```python
from build123d import *

# Parameters (mm, degrees)
SKETCH_2_R               = 72.5
EXTRUDE_1_DEPTH          = 2
CUT_EXTRUDE_1_DEPTH      = 103.549987811
CUT_EXTRUDE_1_DEPTH_BACK = 103.549987811
SKETCH_3_R               = 1.1


with BuildPart() as part:
    # 草图2 → 凸台-拉伸1 (new body)
    with BuildSketch(Plane(origin=(0, 0, 0), x_dir=(1, 0, 0), z_dir=(0, 1, 0))):
        with Locations(Location((0, 0, 0), (0, 0, 270))):
            Circle(SKETCH_2_R)
    extrude(amount=EXTRUDE_1_DEPTH)

    # 草图3 → 切除-拉伸1 (cut, two sides: drawn at the far end of the back side and taken through both)
    with BuildSketch(Plane.XZ.offset(-CUT_EXTRUDE_1_DEPTH_BACK)):
        with Locations(Location((32, 60, 0), (0, 0, 270))):
            Circle(SKETCH_3_R)
        with Locations(Location((-32, 60, 0), (0, 0, 270))):
            Circle(SKETCH_3_R)
        with Locations(Location((-32, -26, 0), (0, 0, 270))):
            Circle(SKETCH_3_R)
        with Locations(Location((32, -26, 0), (0, 0, 270))):
            Circle(SKETCH_3_R)
    extrude(amount=CUT_EXTRUDE_1_DEPTH + CUT_EXTRUDE_1_DEPTH_BACK, mode=Mode.SUBTRACT)


solid = part.part
```
Input: part model. Units: mm. Frame: model coordinates. Give positions to 0.01 mm unless a question says otherwise; leave off trailing zeros. Order: outer loops, then holes, each group sorted by start corner. A loop starts at its lowest first (then second) coordinate and runs counter-clockwise, first axis right, second up.
1. Cut plane A-A (x = -54). Return loops of the section in (y, z).
Computed:
outline: (0, -48.38) - (2, -48.38) - (2, 48.38) - (0, 48.38) - close
2. Cut plane B-B (z = -61.5). Return loops of the section in (x, y), and give its area (3 significant figures).
Computed:
outline: (-38.39, 0) - (38.39, 0) - (38.39, 2) - (-38.39, 2) - close
area: 154 mm2
3. Line query: probe 1 along Z at (x, y) = (-32, 1.1); probe 2 along X at (y, z) = (0.5, -26); probe 3 along X at (y, z) = (0.5, 60). Output: solid intervals per line, ascending.
Computed:
probe 1: z = -65.06 to -27.1, -24.9 to 58.9, 61.1 to 65.06
probe 2: x = -67.68 to -33.1, -30.9 to 30.9, 33.1 to 67.68
probe 3: x = -40.7 to -33.1, -30.9 to 30.9, 33.1 to 40.7
